Geometry: final body of the model. Coordinates: model frame, mm. Face numbers are marked on the shaded views. A direction names the side the tool comes from. Coordinates: 2 decimals unless noted, no trailing zeros. Order: outer loops, then holes, each group sorted by start corner. A loop starts at its lowest first (then second) coordinate and runs counter-clockwise, first axis right, second up. Notation, with made-up numbers: M 43.25,24 L 65.25,24 A28 cw 65.25,58 Z; hole C 56.5,42.5 d3. An arc over 180 degrees is marked long. Write item = value, one per line. Start each with the question number.
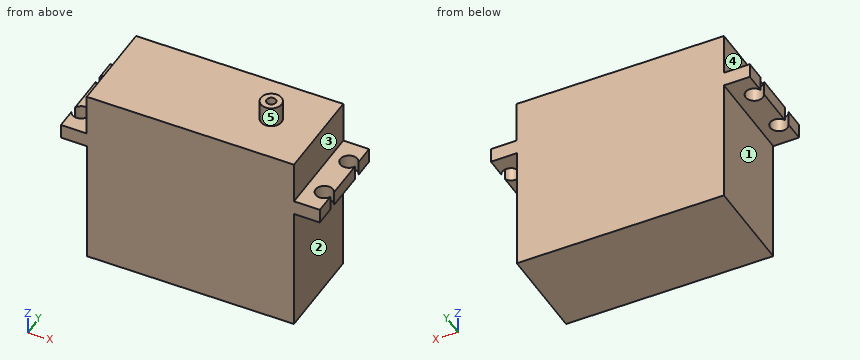
```python
from build123d import *

# Parameters (mm, degrees)
SKETCH_1_W       = 66.04
SKETCH_1_H       = 30.48
EXTRUDE_1_DEPTH  = 40.3754
EXTRUDE_11_DEPTH = 4.64
SKETCH_3_W       = 66.06472
SKETCH_3_H       = 30.48
EXTRUDE_12_DEPTH = 13.462
SKETCH_5_R       = 3.302
SKETCH_5_R_2     = 1.5
EXTRUDE_13_DEPTH = 6.5


with BuildPart() as part:
    # 스케치1 → 보스-돌출1 (new body)
    with BuildSketch(Plane.XY):
        Rectangle(SKETCH_1_W, SKETCH_1_H)
    extrude(amount=EXTRUDE_1_DEPTH)

    # 스케치2 → 보스-돌출11 (add)
    with BuildSketch(Plane.XY.offset(40.3754)):
        with BuildLine():
            Line((41.275, -8.74168445), (41.275, -15.24))
            Line((41.275, -15.24), (-41.275, -15.24))
            Line((-41.275, -15.24), (-41.275, -8.74168445))
            ThreePointArc((-41.275, -8.74168445), (-36.01612, -7.61562), (-41.275, -6.48955555))
            Line((-41.275, -6.48955555), (-41.275, 6.48955555))
            ThreePointArc((-41.275, 6.48955555), (-36.01612, 7.61562), (-41.275, 8.74168445))
            Line((-41.275, 8.74168445), (-41.275, 15.24))
            Line((-41.275, 15.24), (41.275, 15.24))
            Line((41.275, 15.24), (41.275, 8.74168445))
            ThreePointArc((41.275, 8.74168445), (36.01612, 7.61562), (41.275, 6.48955555))
            Line((41.275, 6.48955555), (41.275, -6.48955555))
            ThreePointArc((41.275, -6.48955555), (36.01612, -7.61562), (41.275, -8.74168445))
        make_face()
    extrude(amount=EXTRUDE_11_DEPTH)

    # 스케치3 → 보스-돌출12 (add)
    with BuildSketch(Plane.XY.offset(45.0154)):
        Rectangle(SKETCH_3_W, SKETCH_3_H)
    extrude(amount=EXTRUDE_12_DEPTH)

    # 스케치5 → 보스-돌출13 (add)
    with BuildSketch(Plane.XY.offset(58.4774)):
        with Locations((17.9325, 0)):
            Circle(SKETCH_5_R)
        with Locations((17.9325, 0)):
            Circle(SKETCH_5_R_2, mode=Mode.SUBTRACT)
    extrude(amount=EXTRUDE_13_DEPTH)


solid = part.part
```
Item 1: Reachability of the marked faces 1, 2, 3, 4 and 5 from +Z, -Z, +X, -X, +Y, -Y: full face, straight path, thin tool, end or side. Return the list, or none.
Item 2: Material intervals for probe 1 along Z at (x, y) = (7, 5); probe 2 along X at (y, z) = (1, 25.5); probe 3 along Z at (x, y) = (37.5, -3.5), sorted ascending. Write a range as [from, to].
Item 3: Section query A-A on y = 0. Output: boundary loops of the cut face in (x, z) (1 decimal).
Item 4: First-contact query: pin 1 (9 mm diameter, centred on x = -37.5, y = -4, fed in from +Z); pin 2 (4 mm diameter, centred on y = -6.5, z = 58, fed in from +X); pin 3 (9 mm diameter, centred on x = 38.77, y = -7.62, fed in from +Z). Flat tips, straight axial feed; report the tip coordinate or a pass-through.
Item 5: Section query C-C on z = 32. Output: boundary loops of the cut face in (x, y).
Item 6: Section query B-B on x = 26.5. Output: boundary loops of the cut face in (y, z).
Ans:
q1.face_1 = -Z, -X, +Y, -Y
q1.face_2 = -Z, +X, +Y, -Y
q1.face_3 = +Z, +X, +Y, -Y
q1.face_4 = +Z, -X, +Y, -Y
q1.face_5 = +Z
q2.probe_1 = [0, 58.48]
q2.probe_2 = [-33.02, 33.02]
q2.probe_3 = [40.38, 45.02]
q3.outline = M -41.3,40.4 L -33,40.4 L -33,0 L 33,0 L 33,40.4 L 41.3,40.4 L 41.3,45 L 33,45 L 33,58.5 L 21.2,58.5 L 21.2,65 L 19.4,65 L 19.4,58.5 L 16.4,58.5 L 16.4,65 L 14.6,65 L 14.6,58.5 L -33,58.5 L -33,45 L -41.3,45 Z
q4.pin_1 = 58.48
q4.pin_2 = 33.03
q4.pin_3 = 45.02
q5.outline = M -33.02,-15.24 L 33.02,-15.24 L 33.02,15.24 L -33.02,15.24 Z
q6.outline = M -15.24,0 L 15.24,0 L 15.24,58.48 L -15.24,58.48 Z
